For this review, take the finished solid that the model builds, in its own axes (mm). Round coordinates to 2 decimals unless told otherwise and drop trailing zeros. Order: outer loops, then holes, each group sorted by start corner. A loop starts at its lowest first (then second) coordinate and runs counter-clockwise, first axis right, second up. Notation, with made-up numbers: (4.25, 44) - (8.25, 44) arc R23 ccw to (8.25, 66) - close; hole circle Ø3 at (-40, -38.5). An arc over 180 degrees is marked (long way). Write each question's results on one line, items separated by ' | '. Start each with the question number.
(1) Insertion check: pin 1 Ø3 at (y, z) = (-131, 6) entering from -X; pin 2 Ø6 at (y, z) = (-14, 3) entering from +X; pin 3 Ø1.6 at (y, z) = (-11.5, 3) entering from +X; pin 4 Ø2 at (x, z) = (49.5, 6.5) entering from +Y. Each pin has a flat end and moves straight along its axis. Give the tip position at first contact, or say it passes through.
(2) Take a section at B-B, the plane y = -83. Give the boundary of the cut face in (x, z), plus the area to 3 significant figures.
(3) Take a section at A-A, the plane x = 299. Give the boundary of the cut face in (y, z), plus the area to 3 significant figures.
(4) For L1, parallel to X at y = -142, z = 3.5; L2, parallel to Y at x = 18, z = 5.5; L3, parallel to X at y = -7.5, z = 6.5, list the stretches that pass through material, from the lowest coordinate up. Write a range as from..to.
```python
from build123d import *

# Parameters (mm, degrees)
BOSS_EXTRU_1_DEPTH      = 10
ENL_V_MAT_EXTRU_1_DEPTH = 10
ENL_V_MAT_EXTRU_2_DEPTH = 10
ENL_V_MAT_EXTRU_3_DEPTH = 10


with BuildPart() as part:
    # Esquisse1 → Boss.-Extru.1 (new body)
    with BuildSketch(Plane.XY):
        Polygon((0, 0), (140, 0), (330, -117.424565968), (330, -150), (0, -150), align=None)
    extrude(amount=BOSS_EXTRU_1_DEPTH)

    # Esquisse2 → Enlèv. mat.-Extru.1 (cut)
    with BuildSketch(Plane.XY.offset(10)):
        Polygon((48, -140), (48, -150), (52, -150), (52, -140), (53.55, -140), (53.55, -134.5), (52, -134.5), (52, -128.5), (48, -128.5), (48, -134.5), (46.45, -134.5), (46.45, -140), align=None)
        Polygon((168, -140), (168, -150), (172, -150), (172, -140), (173.55, -140), (173.55, -134.5), (172, -134.5), (172, -128.5), (168, -128.5), (168, -134.5), (166.45, -134.5), (166.45, -140), align=None)
        Polygon((288, -140), (288, -150), (292, -150), (292, -140), (293.55, -140), (293.55, -134.5), (292, -134.5), (292, -128.5), (288, -128.5), (288, -134.5), (286.45, -134.5), (286.45, -140), align=None)
        Polygon((10, -28), (0, -28), (0, -32), (10, -32), (10, -33.55), (15.5, -33.55), (15.5, -32), (21.5, -32), (21.5, -28), (15.5, -28), (15.5, -26.45), (10, -26.45), align=None)
        Polygon((10, -118), (0, -118), (0, -122), (10, -122), (10, -123.55), (15.5, -123.55), (15.5, -122), (21.5, -122), (21.5, -118), (15.5, -118), (15.5, -116.45), (10, -116.45), align=None)
    extrude(amount=-ENL_V_MAT_EXTRU_1_DEPTH, mode=Mode.SUBTRACT)

    # Esquisse3 → Enlèv. mat.-Extru.2 (cut)
    with BuildSketch(Plane.XY.offset(10)):
        Polygon((48, 0), (48, -10), (46.45, -10), (46.45, -15.5), (48, -15.5), (48, -21.5), (52, -21.5), (52, -15.5), (53.55, -15.5), (53.55, -10), (52, -10), (52, 0), align=None)
        Polygon((118, 0), (118, -10), (116.45, -10), (116.45, -15.5), (118, -15.5), (118, -21.5), (122, -21.5), (122, -15.5), (123.55, -15.5), (123.55, -10), (122, -10), (122, 0), align=None)
    extrude(amount=-ENL_V_MAT_EXTRU_2_DEPTH, mode=Mode.SUBTRACT)

    # Esquisse4 → Enlèv. mat.-Extru.3 (cut)
    with BuildSketch(Plane.XY.offset(10)):
        Polygon((180.831420624, -25.234799183), (175.574170795, -33.741345146), (174.25565617, -32.926471422), (171.364168764, -37.605071702), (172.682683388, -38.419945426), (169.528333491, -43.523873004), (172.930951876, -45.626772936), (176.085301774, -40.522845358), (177.403816398, -41.337719081), (180.295303804, -36.659118802), (178.97678918, -35.844245078), (184.23403901, -27.337699114), align=None)
        Polygon((285.76596099, -90.086866854), (280.50871116, -98.593412817), (279.190196536, -97.778539093), (276.29870913, -102.457139373), (277.617223754, -103.272013097), (274.462873856, -108.375940675), (277.865492242, -110.478840607), (281.019842139, -105.374913029), (282.338356764, -106.189786752), (285.22984417, -101.511186473), (283.911329546, -100.696312749), (289.168579376, -92.189766786), align=None)
    extrude(amount=-ENL_V_MAT_EXTRU_3_DEPTH, mode=Mode.SUBTRACT)


solid = part.part
```
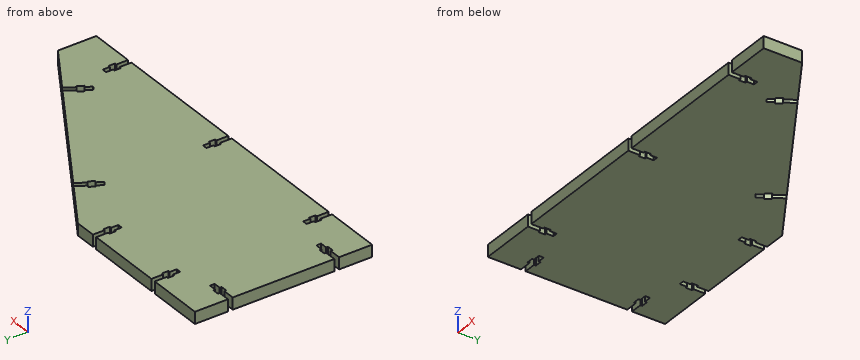
Results below:
1) pin 1: stops at x = 0 | pin 2: stops at x = 167.51 | pin 3: stops at x = 159.9 | pin 4: stops at y = -21.5
2) outline: (0, 0) - (274.3, 0) - (274.3, 10) - (0, 10) - close | area: 2,740 mm^2
3) outline: (-150, 0) - (-98.27, 0) - (-98.27, 10) - (-150, 10) - close | area: 517 mm^2
4) L1: x = 0..48, 52..168, 172..288, 292..330 | L2: y = -150..-122, -118..-32, -28..0 | L3: x = 0..48, 52..118, 122..152.14
